Can you work these out from the model? Positions are in its coordinate system, mm. A direction names the side the tool comes from. Give positions to 0.01 mm unless a question says otherwise; leave off trailing zeros. Loops run counter-clockwise (first coordinate to the right, second up) from the corner with the lowest first, then second, coordinate; pieces in that order, holes last. Notation, with made-up numbers: (54, 31.25) - (69, 31.25) arc R24 cw to (69, 64.25) - close; hole circle Ø10 at (-27.5, -40). An arc over 180 degrees is marked (long way). Answer in a Markdown table with one row per item.
from build123d import *

# Parameters (mm, degrees)
EXTRUDE_1_DEPTH        = 1
CHAMFER_1_SIZE         = 1
CHAMFER_1_SIZE2        = 0.577350269
CHAMFER_1_PART_2_SIZE  = 1
CHAMFER_1_PART_2_SIZE2 = 0.577350269
CHAMFER_1_PART_3_SIZE  = 1
CHAMFER_1_PART_3_SIZE2 = 0.577350269
CHAMFER_1_PART_4_SIZE  = 1
CHAMFER_1_PART_4_SIZE2 = 0.577350269


with BuildPart() as part:
    # Эскиз1 → Бобышка-Вытянуть1 (new body, symmetric)
    with BuildSketch(Plane.XY):
        Polygon((1, 0), (-1, 0), (-1, 5), (-2.75, 5), (-2.75, 6.6), (-2, 6.6), (-2, 21.6), (2, 21.6), (2, 6.6), (2.75, 6.6), (2.75, 5), (1, 5), align=None)
    extrude(amount=EXTRUDE_1_DEPTH, both=True)

    # Фаска1
    chamfer_1_edges = [part.edges().sort_by_distance(p)[0] for p in [
        (0, 21.6, -1),
    ]]
    chamfer_1_side = [part.faces().sort_by_distance(p)[0] for p in [
        (0, 11.701015228, -1),
    ]]
    chamfer(chamfer_1_edges, length=CHAMFER_1_SIZE, length2=CHAMFER_1_SIZE2, reference=chamfer_1_side[0])

    # Фаска1 part 2
    chamfer_1_part_2_edges = [part.edges().sort_by_distance(p)[0] for p in [
        (-2, 21.6, 0),
    ]]
    chamfer_1_part_2_side = [part.faces().sort_by_distance(p)[0] for p in [
        (-2, 14.1, 0),
    ]]
    chamfer(chamfer_1_part_2_edges, length=CHAMFER_1_PART_2_SIZE, length2=CHAMFER_1_PART_2_SIZE2, reference=chamfer_1_part_2_side[0])

    # Фаска1 part 3
    chamfer_1_part_3_edges = [part.edges().sort_by_distance(p)[0] for p in [
        (2, 21.6, 0),
    ]]
    chamfer_1_part_3_side = [part.faces().sort_by_distance(p)[0] for p in [
        (2, 14.1, 0),
    ]]
    chamfer(chamfer_1_part_3_edges, length=CHAMFER_1_PART_3_SIZE, length2=CHAMFER_1_PART_3_SIZE2, reference=chamfer_1_part_3_side[0])

    # Фаска1 part 4
    chamfer_1_part_4_edges = [part.edges().sort_by_distance(p)[0] for p in [
        (0, 21.6, 1),
    ]]
    chamfer_1_part_4_side = [part.faces().sort_by_distance(p)[0] for p in [
        (0, 11.701015228, 1),
    ]]
    chamfer(chamfer_1_part_4_edges, length=CHAMFER_1_PART_4_SIZE, length2=CHAMFER_1_PART_4_SIZE2, reference=chamfer_1_part_4_side[0])


solid = part.part
Q1. Imagine slicing it at D-D, the plane x = 2.3. Write out the boundary of the cut face in (y, z).
Checked values:
| item | result |
|---|---|
| outline | (5, -1) - (6.6, -1) - (6.6, 1) - (5, 1) - close |
Q2. For pin 1 (1 mm diameter, centred on y = 15, z = 0.5, fed in from +X); pin 2 (0.5 mm diameter, centred on x = -2, z = -0.5, fed in from -Y); pin 3 (0.6 mm diameter, centred on x = -2.5, z = 0.5, fed in from +Y), each with a flat end and sliding along its axis, tell me the tip position at first contact or that it passes through.
Checked values:
| item | result |
|---|---|
| pin 1 | stops at x = 2 |
| pin 2 | stops at y = 5 |
| pin 3 | stops at y = 6.6 |
Q3. If we mould it in two halves opening along Z, with no side actions, what happens to faces 5 (the face through (0, 0, 0)), 6 (the face through (0, 10, -1)), 7 (the face through (-0.028, 21.107, 0.707))? For each: released by +Z, released by -Z, zero draft, split by the parting line, or undercut.
Checked values:
| item | result |
|---|---|
| face 5 | zero draft |
| face 6 | released by -Z |
| face 7 | released by +Z |
Q4. Imagine slicing it at A-A, the plane z = 0. Write out the boundary of the cut face in (x, y), and give its area (3 significant figures).
Checked values:
| item | result |
|---|---|
| outline | (-2.75, 5) - (-1, 5) - (-1, 0) - (1, 0) - (1, 5) - (2.75, 5) - (2.75, 6.6) - (2, 6.6) - (2, 20.6) - (1.42, 21.6) - (-1.42, 21.6) - (-2, 20.6) - (-2, 6.6) - (-2.75, 6.6) - close |
| area | 78.2 mm² |
Q5. Imagine slicing it at C-C, the plane y = 7.5. Write out the boundary of the cut face in (x, z), and give its area (3 significant figures).
Checked values:
| item | result |
|---|---|
| outline | (-2, -1) - (2, -1) - (2, 1) - (-2, 1) - close |
| area | 8.00 mm² |
Q6. On a 3-axis mill with a long thin cutter (end or side, diameter ignored), from which of +Z, -Z, +X, -X, +Y, -Y can I reach the whole of each face in a straight line? I mean faces 1 (the face through (1, 3, 0)), 2 (the face through (2, 14, 0)), 3 (the face through (-2, 14, 0)), 4 (the face through (-2, 5, 0)). Say none if no direction works.
Checked values:
| item | result |
|---|---|
| face 1 | +Z, -Z, +X, -Y |
| face 2 | +Z, -Z, +X, +Y |
| face 3 | +Z, -Z, -X, +Y |
| face 4 | +Z, -Z, -X, -Y |
Q7. Imagine slicing it at B-B, the plane x = 1.2. Write out the boundary of the cut face in (y, z), and give its area (3 significant figures).
Checked values:
| item | result |
|---|---|
| outline | (5, -1) - (20.6, -1) - (21.6, -0.42) - (21.6, 0.42) - (20.6, 1) - (5, 1) - close |
| area | 32.6 mm² |
Q8. If I drill on line 1 (X direction, y = 10, z = -0.7); line 2 (X direction, y = 3.75, z = -0.6); line 3 (Y direction, x = -2.4, z = 0.05), over which ranges is the centre line in solid material (lowest first)? Write a range as [from, to].
Checked values:
| item | result |
|---|---|
| line 1 | x = [-2, 2] |
| line 2 | x = [-1, 1] |
| line 3 | y = [5, 6.6] |
